Work out the finished part from the listing and answer in its coordinate system (mm). A direction names the side the tool comes from. Give positions to 0.01 mm unless a question says otherwise; leave off trailing zeros. Loops run counter-clockwise (first coordinate to the right, second up) from the corner with the lowest first, then second, coordinate; pieces in that order, holes last.
from build123d import *

# Parameters (mm, degrees)
CROQUIS2_W              = 6.658935778
CROQUIS2_H              = 6.658935778
CROQUIS2_R              = 1.6
SALIENTE_EXTRUIR1_DEPTH = 1.5
CORTAR_EXTRUIR1_DEPTH   = 1.5


with BuildPart() as part:
    # Croquis1 → Revolución1 (revolve)
    with BuildSketch(Plane.XY, mode=Mode.PRIVATE) as revoluci_n1_sk:
        Polygon((1.6, 0), (7, 0), (7, 3), (4.85, 3), (4.85, 8.4), (1.6, 8.4), align=None)
    revolve(revoluci_n1_sk.sketch.rotate(Axis((0, -1000, 0), (0, 1, 0)), 90), axis=Axis((0, -1000, 0), (0, 1, 0)))

    # Croquis2 → Saliente-Extruir1 (add)
    with BuildSketch(Plane(origin=(0, 8.4, 0), x_dir=(1, 0, 0), z_dir=(0, 1, 0))):
        Rectangle(CROQUIS2_W, CROQUIS2_H)
        with Locations(Location((0, 0, 0), (0, 0, 90))):
            Circle(CROQUIS2_R, mode=Mode.SUBTRACT)
    extrude(amount=SALIENTE_EXTRUIR1_DEPTH)

    # Croquis3 → Cortar-Extruir1 (cut)
    with BuildSketch(Plane(origin=(0, 0, 0), x_dir=(1, 0, 0), z_dir=(0, 1, 0))):
        Polygon((4.65, 0), (2.325, 4.027018128), (-2.325, 4.027018128), (-4.65, 0), (-2.325, -4.027018128), (2.325, -4.027018128), align=None)
    extrude(amount=CORTAR_EXTRUIR1_DEPTH, mode=Mode.SUBTRACT)


solid = part.part
Item 1: For faces 5 (the face through (3.329, 9, 0)), 6 (the face through (0, 9, 3.329)), 7 (the face through (4.3, 5.74, -2.24)), 8 (the face through (3.5, 0.74, -1.99)), 9 (the face through (0, 9, -3.329)), determine the directions among +Z, -Z, +X, -X, +Y, -Y from which every point of the face is accessible in a straight line to the end or side of a thin tool.
Item 2: Find section C-C, the plane y = 6. Write down the section's boundary in (x, z).
Item 3: Find section B-B, the plane x = 0. Write down the section's boundary in (y, z).
Item 4: Determine the mould class of faces 1 (the face through (-3.329, 9, 0)), 2 (the face through (0, 1, 4.027)), 3 (the face through (2, 1.5, 0)), 4 (the face through (-2, 9.9, -1)) for opening direction X: released by +X, released by -X, zero draft, split by the parting line, or undercut.
Item 5: Flat-ended cylindrical pins translate along their axes: pin 1 Ø1.2 at (x, y) = (1, 1) entering from -Z; pin 2 Ø1.6 at (x, y) = (0, 9.5) entering from -Z; pin 3 Ø3 at (y, z) = (8, 3.5) entering from +X; pin 4 Ø8 at (x, z) = (-3.5, -4) entering from -Y. Find the tip coordinate at first contact, or state that the pin passes through.
Item 6: Consider line 1 (X direction, y = 6.25, z = 0); line 2 (Y direction, x = 0.5, z = 6.25); line 3 (Y direction, x = -3.5, z = -3). Determine where each line is inside the solid, lowest interval first.
Item 7: Find section A-A, the plane z = -1.25. Write down the section's boundary in (x, y).
Item 8: Find section D-D, the plane x = -4. Write down the section's boundary in (y, z), plus the area to 3 significant figures.
Ans:
1. face 5: +Z, -Z, +X, +Y
1. face 6: +Z, +X, -X, +Y
1. face 7: +Y
1. face 8: -Y
1. face 9: -Z, +X, -X, +Y
2. outline: circle Ø9.7 at (0, 0); hole circle Ø3.2 at (0, 0)
3. outline: (0, -7) - (3, -7) - (3, -4.85) - (8.4, -4.85) - (8.4, -3.33) - (9.9, -3.33) - (9.9, -1.6) - (1.5, -1.6) - (1.5, -4.03) - (0, -4.03) - close; (0, 4.03) - (1.5, 4.03) - (1.5, 1.6) - (9.9, 1.6) - (9.9, 3.33) - (8.4, 3.33) - (8.4, 4.85) - (3, 4.85) - (3, 7) - (0, 7) - close
4. face 1: released by -X
4. face 2: undercut
4. face 3: undercut
4. face 4: zero draft
5. pin 1: stops at z = -6.99
5. pin 2: stops at z = -3.33
5. pin 3: stops at x = 4.42
5. pin 4: stops at y = 0
6. line 1: x = -4.85 to -1.6, 1.6 to 4.85
6. line 2: y = 0 to 3
6. line 3: y = 0 to 8.4
7. outline: (-6.89, 0) - (-3.93, 0) - (-3.93, 1.5) - (-1, 1.5) - (-1, 9.9) - (-3.33, 9.9) - (-3.33, 8.4) - (-4.69, 8.4) - (-4.69, 3) - (-6.89, 3) - close; (1, 1.5) - (3.93, 1.5) - (3.93, 0) - (6.89, 0) - (6.89, 3) - (4.69, 3) - (4.69, 8.4) - (3.33, 8.4) - (3.33, 9.9) - (1, 9.9) - close
8. outline: (0, -5.74) - (3, -5.74) - (3, -2.74) - (8.4, -2.74) - (8.4, 2.74) - (3, 2.74) - (3, 5.74) - (0, 5.74) - (0, 1.13) - (1.5, 1.13) - (1.5, -1.13) - (0, -1.13) - close
8. area: 60.7 mm2
